```python
from build123d import *

# Parameters (mm, degrees)
SKETCH_W             = 18
SKETCH_H             = 19.2
PAD_DEPTH            = 4
POCKET_DEPTH         = 0.001
POCKET_DEPTH_BACK    = -4.001
POCKET001_DEPTH      = 0.001
POCKET001_DEPTH_BACK = -18.001
SKETCH003_R          = 5
POCKET002_DEPTH      = 4.001


with BuildPart() as part:
    # Sketch → Pad (new body)
    with BuildSketch(Plane.XY):
        with Locations((9, 9.6)):
            Rectangle(SKETCH_W, SKETCH_H)
    extrude(amount=PAD_DEPTH)

    # Sketch001 → Pocket (cut, two sides)
    with BuildSketch(Plane.XY) as pocket_sk:
        with BuildLine():
            ThreePointArc((3.3, 11.35), (2.75, 11.9), (2.2, 11.35))
            Line((2.2, 11.35), (2.2, 7.85))
            ThreePointArc((2.2, 7.85), (2.75, 7.3), (3.3, 7.85))
            Line((3.3, 7.85), (3.3, 11.35))
        make_face()
        with BuildLine():
            ThreePointArc((15.8, 11.35), (15.25, 11.9), (14.7, 11.35))
            Line((14.7, 11.35), (14.7, 7.85))
            ThreePointArc((14.7, 7.85), (15.25, 7.3), (15.8, 7.85))
            Line((15.8, 7.85), (15.8, 11.35))
        make_face()
        with BuildLine():
            ThreePointArc((5.5, 16.6), (6.5, 15.6), (7.5, 16.6))
            Line((7.5, 16.6), (7.5, 17.6))
            ThreePointArc((7.5, 17.6), (6.5, 18.6), (5.5, 17.6))
            Line((5.5, 17.6), (5.5, 16.6))
        make_face()
        with BuildLine():
            ThreePointArc((10.5, 16.6), (11.5, 15.6), (12.5, 16.6))
            Line((12.5, 16.6), (12.5, 17.6))
            ThreePointArc((12.5, 17.6), (11.5, 18.6), (10.5, 17.6))
            Line((10.5, 17.6), (10.5, 16.6))
        make_face()
        with BuildLine():
            ThreePointArc((12.5, 2.6), (11.5, 3.6), (10.5, 2.6))
            Line((10.5, 2.6), (10.5, 1.6))
            ThreePointArc((10.5, 1.6), (11.5, 0.6), (12.5, 1.6))
            Line((12.5, 1.6), (12.5, 2.6))
        make_face()
        with BuildLine():
            ThreePointArc((10, 2.6), (9, 3.6), (8, 2.6))
            Line((8, 2.6), (8, 1.6))
            ThreePointArc((8, 1.6), (9, 0.6), (10, 1.6))
            Line((10, 1.6), (10, 2.6))
        make_face()
        with BuildLine():
            ThreePointArc((7.5, 2.6), (6.5, 3.6), (5.5, 2.6))
            Line((5.5, 2.6), (5.5, 1.6))
            ThreePointArc((5.5, 1.6), (6.5, 0.6), (7.5, 1.6))
            Line((7.5, 1.6), (7.5, 2.6))
        make_face()
    extrude(amount=-POCKET_DEPTH, mode=Mode.SUBTRACT)
    extrude(pocket_sk.sketch, amount=-POCKET_DEPTH_BACK, mode=Mode.SUBTRACT)

    # Sketch002 → Pocket001 (cut, two sides)
    with BuildSketch(Plane.YZ) as pocket001_sk:
        with BuildLine():
            ThreePointArc((7.85, 3), (6.85, 2), (7.85, 1))
            Line((7.85, 1), (11.35, 1))
            ThreePointArc((11.35, 1), (12.35, 2), (11.35, 3))
            Line((11.35, 3), (7.85, 3))
        make_face()
    extrude(amount=-POCKET001_DEPTH, mode=Mode.SUBTRACT)
    extrude(pocket001_sk.sketch, amount=-POCKET001_DEPTH_BACK, mode=Mode.SUBTRACT)

    # Sketch003 (on DatumPlane) → Pocket002 (cut, through all)
    with BuildSketch(Plane.XY.offset(4)):
        with Locations((9, 9.6)):
            Circle(SKETCH003_R)
    extrude(amount=-POCKET002_DEPTH, mode=Mode.SUBTRACT)


solid = part.part
```
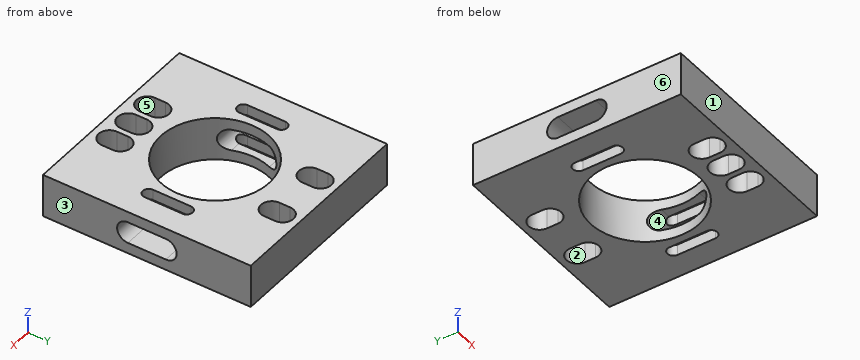
Verification items for the finished model (mm, model axes). Face numbers are marked on the shaded views. A direction names the side the tool comes from. Coordinates: 2 decimals unless noted, no trailing zeros. Loops run counter-clockwise (first coordinate to the right, second up) from the corner with the lowest first, then second, coordinate; pieces in that order, holes last. Notation, with made-up numbers: (53, -33.5) -> (109, -33.5) arc R23 cw to (109, 3.5) -> close; hole circle Ø8 at (20.25, -34). An arc over 180 degrees is marked (long way). Answer in a Markdown table with one row per item.
1) Draft check along Y on the marked faces 1, 2 and 3. Enter one of: released by +Y, released by -Y, zero draft, split by the parting line, or undercut.
The answers:
| item | result |
|---|---|
| face 1 | released by -Y |
| face 2 | undercut |
| face 3 | zero draft |
2) Section check A-A (z = 2). Give the number of separate pieces and of enclosed holes in the cut face, and give its area (3 significant figures).
The answers:
| item | result |
|---|---|
| separate pieces | 2 |
| enclosed holes | 5 |
| area | 194 mm2 |
3) Access from +Z, -Z, +X, -X, +Y, -Y to the whole of each face (thin tool, end or side, straight path). Record for the marked faces 4, 5 and 6.
The answers:
| item | result |
|---|---|
| face 4 | +X, -X |
| face 5 | +Z, -Z |
| face 6 | +Z, -Z, -X, +Y, -Y |
4) Section check C-C (x = 1). Record the cut outline in (y, z), and give its area (3 significant figures).
The answers:
| item | result |
|---|---|
| outline | (0, 0) -> (19.2, 0) -> (19.2, 4) -> (0, 4) -> close; hole (7.85, 1) -> (11.35, 1) arc R1 ccw to (11.35, 3) -> (7.85, 3) arc R1 ccw to start |
| area | 66.7 mm2 |
5) Section check B-B (y = 17.25). Record the cut outline in (x, z).
The answers:
| item | result |
|---|---|
| outline | (0, 0) -> (5.5, 0) -> (5.5, 4) -> (0, 4) -> close; (7.5, 0) -> (10.5, 0) -> (10.5, 4) -> (7.5, 4) -> close; (12.5, 0) -> (18, 0) -> (18, 4) -> (12.5, 4) -> close |
6) Scan lines: line 1 along Y through (x, z) = (9, 1.3); line 2 along X through (y, z) = (2.5, 1.2); line 3 along Y through (x, z) = (6.5, 2.6). Record each from-to range of solid material in increasing order. Write a range as from..to.
The answers:
| item | result |
|---|---|
| line 1 | y = 0..0.6, 3.6..4.6, 14.6..19.2 |
| line 2 | x = 0..5.5, 7.5..8, 10..10.5, 12.5..18 |
| line 3 | y = 0..0.6, 3.6..5.27, 13.93..15.6, 18.6..19.2 |
